Autodesk Inventor part; units mm, degrees
ref_plane "YZ Plane" through (0, 0, 0) normal (1, 0, 0) x (0, 1, 0)
ref_plane "XZ Plane" through (0, 0, 0) normal (0, 1, 0) x (-1, 0, 0)
ref_plane "XY Plane" through (0, 0, 0) normal (0, 0, 1) x (1, 0, 0)
sketch "Sketch1" plane through (0, 0, 0) normal (0, 0, 1) x (1, 0, 0)
  line L0 (-7.5, -7.5) -> (7.5, -7.5)
  line L1 (7.5, -7.5) -> (7.5, 7.5)
  line L2 (7.5, 7.5) -> (-7.5, 7.5)
  line L3 (-7.5, 7.5) -> (-7.5, -7.5)
  line L4 (-7.5, -7.5) -> (7.5, 7.5) construction
  line L5 (7.5, -7.5) -> (-7.5, 7.5) construction
  point P0 (0, 0)
  dimension "d0" = 15
  dimension "d1" = 15
extrude "Extrusion1" add sketch "Sketch1" along normal blind 133
ref_plane "Work Plane1" through (0, 0, 66.5) normal (0, 0, 1) x (1, 0, 0)
sketch "Sketch2" plane through (0, 0, 133) normal (0, 0, 1) x (1, 0, 0)
  line L0 (-5, -5) -> (5, -5)
  line L1 (5, -5) -> (5, 5)
  line L2 (5, 5) -> (-5, 5)
  line L3 (-5, 5) -> (-5, -5)
  line L4 (-5, -5) -> (5, 5) construction
  line L5 (5, -5) -> (-5, 5) construction
  point P0 (0, 0)
  dimension "d4" = 10
  dimension "d5" = 10
extrude "Extrusion2" add sketch "Sketch2" along normal blind 14
mirror "Mirror1" about plane through (0, 0, 66.5) normal (0, 0, 1) of "Extrusion2"
sketch "Sketch3" plane through (0, 0, 147) normal (0, 0, 1) x (1, 0, 0)
  line L0 (-5, -5) -> (5, -5)
  line L1 (5, -5) -> (5, 5)
  line L2 (5, 5) -> (-5, 5)
  line L3 (-5, 5) -> (-5, -5)
  line L4 (-4.6, -4.6) -> (4.6, -4.6)
  line L5 (4.6, -4.6) -> (4.6, 4.6)
  line L6 (4.6, 4.6) -> (-4.6, 4.6)
  line L7 (-4.6, 4.6) -> (-4.6, -4.6)
  point P0 (0, 0)
  dimension "d8" = 0.4
extrude "Extrusion3" cut sketch "Sketch3" against normal up to surface (14 mm away)
mirror "Mirror2" about plane through (0, 0, 66.5) normal (0, 0, 1) of "Extrusion2"
mirror "Mirror3" about plane through (0, 0, 66.5) normal (0, 0, 1) of "Extrusion3"
properties part number "Upper Beam Support"
The listing builds one solid part. Answer for the finished solid, in the listing's coordinates (mm). A direction names the side the tool comes from. Coordinates: 2 decimals unless noted, no trailing zeros. Write each loop counter-clockwise with the first axis right and the second up, starting at its lowest first coordinate (ties: lowest second). Pieces come first, ordered by that corner, then holes. Notation, with made-up numbers: M 65,-17 L 72,-17 A32 ccw 72,17 Z; hole C 83.5,-13 d3. An arc over 180 degrees is marked long. Write each question's results on one line, items separated by ' | '.
Item 1: Which of the six approach directions +Z, -Z, +X, -X, +Y, -Y give full straight-line access (tool end or side, diameter ignored) to faces 1 (the face through (0, 4.6, 140)), 2 (the face through (4.6, 0, 140)), 3 (the face through (4.6, 0, -7)), 4 (the face through (0, 4.6, -7))?
Answer below:
face 1: +Z, +X, -X, +Y | face 2: +Z, +X, +Y, -Y | face 3: -Z, +X, +Y, -Y | face 4: -Z, +X, -X, +Y
Item 2: Given P1, Ø3, axis at y = 0.5, z = -5, coming from the +X side; P2, Ø7.5, axis at x = 0.5, z = 140.5, coming from the +Y side; P3, Ø3, axis at y = 1, z = -8.5, coming from the -X side, each flat-ended and moving along its own axis, determine where each tip first touches the part or whether it passes through.
Answer below:
P1: x = 4.6 | P2: y = 4.6 | P3: x = -4.6
Item 3: Consider probe 1 along Y at (x, z) = (-3.25, -6.5); probe 2 along Z at (x, y) = (6.25, -2). Determine where each line is inside the solid, lowest interval first. Write a range as [from, to].
Answer below:
probe 1: [-4.6, 4.6] | probe 2: [0, 133]
Item 4: The part is cut by section A-A on y = 1. Determine the outline of the cut face in (x, z).
Answer below:
outline: M -7.5,0 L -4.6,0 L -4.6,-14 L 4.6,-14 L 4.6,0 L 7.5,0 L 7.5,133 L 4.6,133 L 4.6,147 L -4.6,147 L -4.6,133 L -7.5,133 Z
